from build123d import *

# Parameters (mm, degrees)
SKETCH1_W              = 5.75
SKETCH1_H              = 330
BOSS_EXTRUDE1_DEPTH    = 60
CUT_EXTRUDE1_START     = -5.75
CUT_EXTRUDE1_OUTLINE_R = 11
CUT_EXTRUDE1_DEPTH     = 5.75
M4_CLEARANCE_HOLE1_D   = 4.5
SKETCH10_R             = 11.1125
CUT_EXTRUDE4_DEPTH     = 5.75
SKETCH13_R             = 6
SKETCH13_W             = 20
SKETCH13_H             = 150
CUT_EXTRUDE5_DEPTH     = 5.75
FILLET2_R              = 3
M3_CLEARANCE_HOLE1_D   = 3.4


# Read off the part's stored shape, not the designer's step: Cut-Extrude1
with BuildPart() as part:
    # Sketch1 → Boss-Extrude1 (new body)
    with BuildSketch(Plane(origin=(0, 0, 0), x_dir=(0, 0, -1), z_dir=(1, 0, 0))):
        with Locations((-2.875, 165)):
            Rectangle(SKETCH1_W, SKETCH1_H)
    extrude(amount=BOSS_EXTRUDE1_DEPTH)

    # Cut-Extrude1 outline → Cut-Extrude1 (cut)
    with BuildSketch(Plane.XY.offset(5.75).offset(CUT_EXTRUDE1_START)):
        with BuildLine():
            ThreePointArc((0, 300), (8.786796564, 321.213203436), (30, 330))
            Line((30, 330), (0, 330))
            Line((0, 330), (0, 300))
        make_face()
        with BuildLine():
            ThreePointArc((30, 330), (51.213203436, 321.213203436), (60, 300))
            Line((60, 300), (60, 330))
            Line((60, 330), (30, 330))
        make_face()
        with Locations((30, 300)):
            Circle(CUT_EXTRUDE1_OUTLINE_R)
    extrude(amount=CUT_EXTRUDE1_DEPTH, mode=Mode.SUBTRACT)

    # M4 Clearance Hole1 (through all)
    with Locations(Plane.XY.offset(5.75)):
        with Locations((19.393398282, 310.606601718), (40.606601718, 310.606601718), (40.606601718, 289.393398282), (19.393398282, 289.393398282)):
            Hole(M4_CLEARANCE_HOLE1_D / 2)

    # Sketch10 → Cut-Extrude4 (cut)
    with BuildSketch(Plane(origin=(0, 0, 0), x_dir=(-1, 0, 0), z_dir=(0, 0, -1))):
        with Locations(Location((-30, 14, 0), (0, 0, 90))):
            Circle(SKETCH10_R)
    extrude(amount=-CUT_EXTRUDE4_DEPTH, mode=Mode.SUBTRACT)

    # Sketch13 → Cut-Extrude5 (cut)
    with BuildSketch(Plane(origin=(0, 0, 0), x_dir=(-1, 0, 0), z_dir=(0, 0, -1))):
        with Locations(Location((-30, 60, 0), (0, 0, 90))):
            Circle(SKETCH13_R)
        with Locations((-40, 175)):
            Rectangle(SKETCH13_W, SKETCH13_H)
        with BuildLine():
            Line((-60, 285.857864376), (-60, 300))
            ThreePointArc((-60, 300), (-59.277002188, 306.546536707), (-57.142857143, 312.7775313))
            ThreePointArc((-57.142857143, 312.7775313), (-50.08377905, 298.416853586), (-60, 285.857864376))
        make_face()
    extrude(amount=-CUT_EXTRUDE5_DEPTH, mode=Mode.SUBTRACT)

    # Fillet2
    fillet2_edges = [part.edges().sort_by_distance(p)[0] for p in [
        (60, 0, 2.875),
        (0, 0, 2.875),
        (57.142857143, 312.7775313, 2.875),
        (60, 285.857864376, 2.875),
        (50, 100, 2.875),
        (50, 250, 2.875),
        (30, 250, 2.875),
        (30, 100, 2.875),
    ]]
    fillet(fillet2_edges, radius=FILLET2_R)

    # M3 Clearance Hole1 (through all)
    with Locations(Plane(origin=(0, 0, 0), x_dir=(-1, 0, 0), z_dir=(0, 0, -1))):
        with Locations((-11.50000102, 240.99999992), (-55.00000038, 240.99999992), (-11.50000102, 105.49999914), (-55.00000038, 105.49999914), (-5, 160), (-26.4, 199.7)):
            Hole(M3_CLEARANCE_HOLE1_D / 2)


solid = part.part
Design review of the part built by this model. Coordinates are the model's own, in mm. A direction names the side the tool comes from. Give positions to 0.01 mm unless a question says otherwise; leave off trailing zeros. Write each loop counter-clockwise with the first axis right and the second up, starting at its lowest first coordinate (ties: lowest second). Pieces come first, ordered by that corner, then holes. Notation, with made-up numbers: M 1.25,-7.5 L 18.25,-7.5 A13 ccw 18.25,11.5 Z; hole C 49.5,84.5 d2. An arc over 180 degrees is marked long. Return JSON: item names as keys, results as strings. Group by question number.
Item 1: Clearance check with a flat-ended pin moving along its axis: pin 1 Ø3 at (x, y) = (55, 241) entering from -Z. State where the tip first meets the part, or that it passes through.
Item 2: Take a section at B-B (y = 296.5). Give the boundary of the cut face in (x, z), plus the area to 3 significant figures.
Item 3: The part is to be moulded in two halves that separate along Y. For faces 3 (the flat face through (0, 154, 3)), 4 (the flat face through (40, 250, 3)), 5 (the flat face through (30, 0, 3)), say which applies: pulls with the +Y half, pulls with the -Y half, needs draft (parallel to the pull), parting line crosses it, or undercut.
Item 4: Tool access review of faces 1 (the flat face through (30, 174, 3)), 2 (the cylindrical face through (50.09, 298.35, 2.83)): name each direction out of +Z, -Z, +X, -X, +Y, -Y from which nothing blocks a thin tool from reaching the whole face with its end or side.
Item 5: Take a section at C-C (z = 2.1). Count the separate pieces of the cut face and the enclosed holes in it, plus the area to 3 significant figures.
Item 6: Take a section at A-A (y = 230.5). Give the boundary of the cut face in (x, z), plus the area to 3 significant figures.
Item 7: Wall thickness on line 1 along X through (y, z) = (160, 3.35); line 2 along X through (y, z) = (167, 0.75); line 3 along X through (y, z) = (199, 3.55): over which ranges is each line inside the solid? List them lowest first.
Return value:
{
 "1": {"pin 1": "passes through"},
 "2": {"outline": "M 0,0 L 19.57,0 L 19.57,5.75 L 0,5.75 Z; M 40.43,0 L 50.41,0 L 50.41,5.75 L 40.43,5.75 Z", "area": "170 mm2"},
 "3": {"face 3": "needs draft", "face 4": "undercut", "face 5": "pulls with the -Y half"},
 "4": {"face 1": "+Z, -Z", "face 2": "+Z, -Z, +X"},
 "5": {"separate pieces": "1", "enclosed holes": "14", "area": "15,200 mm2"},
 "6": {"outline": "M 0,0 L 30,0 L 30,5.75 L 0,5.75 Z; M 50,0 L 60,0 L 60,5.75 L 50,5.75 Z", "area": "230 mm2"},
 "7": {"line 1": "x = 0 to 3.3, 6.7 to 30, 50 to 60", "line 2": "x = 0 to 30, 50 to 60", "line 3": "x = 0 to 24.85, 27.95 to 30, 50 to 60"}
}
